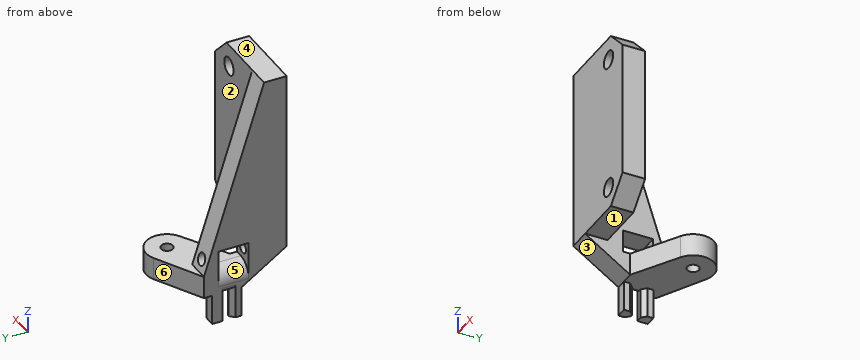
from build123d import *

# Parameters (mm, degrees)
SKETCH1_W                    = 12.192
SKETCH1_H                    = 30.62
SKETCH1_R                    = 1.5
BOSS_EXTRUDE1_DEPTH          = 3.81
BOSS_EXTRUDE2_DEPTH          = 3.81
SKETCH3_W                    = 1.778
SKETCH3_H                    = 1.778
BOSS_EXTRUDE3_DEPTH          = 5.08
SKETCH4_R                    = 1
BOSS_EXTRUDE4_DEPTH          = 3.81
CUT_EXTRUDE1_REACH           = 18.002
SKETCH5_W                    = 3.81
SKETCH5_H                    = 5.08
SKETCH6_R                    = 1
CUT_EXTRUDE2_DEPTH           = 13.310347601
CUT_EXTRUDE2_OTHER_WAY_DEPTH = 5.08
CUT_EXTRUDE2_OTHER_WAY_TAPER = 5
CHAMFER1_SIZE                = 0.762
FILLET1_R                    = 2.54
CHAMFER2_SIZE                = 3.81
FILLET2_R                    = 0.762


with BuildPart() as part:
    # Sketch1 → Boss-Extrude1 (new body)
    with BuildSketch(Plane(origin=(0, 0, 0), x_dir=(1, 0, 0), z_dir=(0, 1, 0))):
        with Locations((6.096, 15.31)):
            Rectangle(SKETCH1_W, SKETCH1_H)
        with Locations((7.62, 26.81)):
            Circle(SKETCH1_R, mode=Mode.SUBTRACT)
        with Locations((7.62, 3.81)):
            Circle(SKETCH1_R, mode=Mode.SUBTRACT)
    extrude(amount=BOSS_EXTRUDE1_DEPTH)

    # Sketch2 → Boss-Extrude2 (add)
    with BuildSketch(Plane.ZY):
        Polygon((0, 3.81), (0, 0), (-30.62, 0), (-35.7, 7.62), (-35.7, 13.97), (-31.89, 13.97), align=None)
    extrude(amount=BOSS_EXTRUDE2_DEPTH)

    # Sketch3 → Boss-Extrude3 (add)
    with BuildSketch(Plane(origin=(0, 0, -35.7), x_dir=(-1, 0, 0), z_dir=(0, 0, -1))):
        with Locations((2.921, 8.509)):
            Rectangle(SKETCH3_W, SKETCH3_H)
        with Locations((2.921, 11.684)):
            Rectangle(SKETCH3_W, SKETCH3_H)
    extrude(amount=BOSS_EXTRUDE3_DEPTH)

    # Sketch4 → Boss-Extrude4 (add)
    with BuildSketch(Plane(origin=(0, 0, -35.7), x_dir=(-1, 0, 0), z_dir=(0, 0, -1))):
        with BuildLine():
            Line((0, 7.62), (-7.670279519, 12.123848354))
            ThreePointArc((-7.670279519, 12.123848354), (-8.962218829, 16.913759957), (-4.196321779, 18.2916517))
            Line((-4.196321779, 18.2916517), (3.81, 13.97))
            Line((3.81, 13.97), (0, 13.97))
            Line((0, 13.97), (0, 7.62))
        make_face()
        with Locations((-5.877818102, 15.1765)):
            Circle(SKETCH4_R, mode=Mode.SUBTRACT)
    extrude(amount=-BOSS_EXTRUDE4_DEPTH)

    # Sketch5 → Cut-Extrude1 (cut, up to next)
    with BuildSketch(Plane.ZY.offset(3.81), mode=Mode.PRIVATE) as cut_extrude1_sk1:
        with Locations((-29.985, 8.946152399)):
            Rectangle(SKETCH5_W, SKETCH5_H)
    cut_extrude1_tool1 = extrude(cut_extrude1_sk1.sketch, amount=-CUT_EXTRUDE1_REACH, mode=Mode.PRIVATE) & part.part
    add(cut_extrude1_tool1.solids().sort_by_distance((-3.81, 8.946152, -29.985))[0], mode=Mode.SUBTRACT)

    # Sketch6 → Cut-Extrude2 (cut)
    with BuildSketch(Plane(origin=(0, 6.406152399, 0), x_dir=(1, 0, 0), z_dir=(0, 1, 0))):
        with Locations((-1.905, 29.985)):
            Circle(SKETCH6_R)
    extrude(amount=CUT_EXTRUDE2_DEPTH, mode=Mode.SUBTRACT)

    # Sketch6 → Cut-Extrude2 other way (cut)
    with BuildSketch(Plane(origin=(0, 6.406152399, 0), x_dir=(1, 0, 0), z_dir=(0, 1, 0))):
        with Locations((-1.905, 29.985)):
            Circle(SKETCH6_R)
    extrude(amount=-CUT_EXTRUDE2_OTHER_WAY_DEPTH, taper=CUT_EXTRUDE2_OTHER_WAY_TAPER, mode=Mode.SUBTRACT)

    # Chamfer1
    chamfer1_edges = [part.edges().sort_by_distance(p)[0] for p in [
        (-3.81, 9.398, -38.24),
        (-2.032, 9.398, -38.24),
        (-2.032, 10.795, -38.24),
    ]]
    chamfer(chamfer1_edges, length=CHAMFER1_SIZE)

    # Fillet1
    fillet1_edges = [part.edges().sort_by_distance(p)[0] for p in [
        (-3.81, 8.946152399, -31.89),
    ]]
    fillet(fillet1_edges, radius=FILLET1_R)

    # Chamfer2
    chamfer2_edges = [part.edges().sort_by_distance(p)[0] for p in [
        (12.192, 1.905, -30.62),
        (12.192, 1.905, 0),
    ]]
    chamfer(chamfer2_edges, length=CHAMFER2_SIZE)

    # Fillet2
    fillet2_edges = [part.edges().sort_by_distance(p)[0] for p in [
        (-3.81, 10.0965, -35.7),
    ]]
    fillet(fillet2_edges, radius=FILLET2_R)


solid = part.part
Input: part model. Units: mm. Frame: model coordinates. Face numbers are marked on the shaded views. A direction names the side the tool comes from. Give positions to 0.01 mm unless a question says otherwise; leave off trailing zeros. Write each loop counter-clockwise with the first axis right and the second up, starting at its lowest first coordinate (ties: lowest second). Pieces come first, ordered by that corner, then holes.
Q1. Section A-A, the plane y = 10. Output: boundary loops of the cut face in (x, z).
Q2. Section D-D, the plane y = 5.5. Output: boundary loops of the cut face in (x, z) (3 decimals), plus the area to 3 significant figures.
Q3. Material intervals for probe 1 along Z at (x, y) = (7.62, 1.5); probe 2 along X at (y, z) = (1, -3.81); probe 3 along Y at (x, z) = (6, -11), sorted ascending.
Q4. Set-up query: the marked faces 1, 2 and 3. Return all of +Z, -Z, +X, -X, +Y, -Y with unobstructed straight access to the full face (end or side cutting, diameter ignored); none if empty.
Q5. Pull-direction query (Y, two-part tool) for the marked faces 4, 5 and 6; classes: pulls with the +Y half, pulls with the -Y half, needs draft (parallel to the pull), parting line crosses it, or undercut.
Q6. Section B-B, the plane z = -3. Output: boundary loops of the cut face in (x, y), plus the area to 3 significant figures.
Q7. First-contact query: P1, Ø0.5, axis at x = -3.5, z = -38, coming from the -Y side; P2, Ø6, axis at x = 10, y = 3, coming from the -Z side; P3, Ø0.8, axis at y = 12, z = -37.5, coming from the +X side. Flat tips, straight axial feed; report the tip coordinate or a pass-through.
Filled in:
1. outline: (-3.81, -34.94) arc R0.76 ccw to (-3.05, -35.7) - (4.05, -35.7) - (4.05, -31.89) - (-1.27, -31.89) arc R2.54 ccw to (-3.81, -34.43) - close; (-3.81, -28.08) - (0, -28.08) - (0, -19.43) - (-3.81, -19.43) - close
2. outline: (-3.81, -34.287) - (0, -34.287) - (0, -5.305) - (-3.81, -5.305) - close; hole circle Ø1.841 at (-1.905, -29.985)
2. area: 108 mm2
3. probe 1: z = -30.62 to -28.31, -25.31 to -5.31, -2.31 to 0
3. probe 2: x = -3.81 to 6.12, 9.12 to 12.19
3. probe 3: y = 0 to 3.81
4. face 1: -Z, +X, +Y, -Y
4. face 2: +Z, -Z, +X, +Y
4. face 3: -Z, +X, -X, -Y
5. face 4: needs draft
5. face 5: undercut
5. face 6: pulls with the +Y half
6. outline: (-3.81, 0) - (6.36, 0) - (6.36, 3.81) - (0, 3.81) - (0, 4.77) - (-3.81, 4.77) - close; (8.88, 0) - (11.38, 0) - (11.38, 3.81) - (8.88, 3.81) - close
6. area: 51.9 mm2
7. P1: stops at y = 7.62
7. P2: stops at z = -30.62
7. P3: stops at x = -2.03
